Autodesk Inventor part; units mm, degrees
ref_plane "YZ Plane" through (0, 0, 0) normal (1, 0, 0) x (0, 1, 0)
ref_plane "XZ Plane" through (0, 0, 0) normal (0, 1, 0) x (-1, 0, 0)
ref_plane "XY Plane" through (0, 0, 0) normal (0, 0, 1) x (1, 0, 0)
sketch "Sketch_1" plane through (0, 0, 0) normal (0, 0, 1) x (1, 0, 0)
  line L0 (11, 0) -> (-2.8, 0)
  line L1 (-2.8, 0) -> (-2.8, 5)
  line L2 (-2.8, 5) -> (0, 5)
  line L3 (0, 5) -> (0, 3)
  line L4 (0, 3) -> (11, 3)
  line L5 (11, 3) -> (11, 0)
  line L6 (11, 0) -> (-2.8, 0)
revolve "Revolution1" add sketch "Sketch_1" angle 360 about axis through (11, 0, 0) along (1, 0, 0)
sketch "Sketch2" plane through (-2.8, 0, 0) normal (-1, 0, 0) x (0, 0, 1)
  point P0 (0, 0)
hole "Hole1" at (-2.8, 0, 0) direction (1, 0, 0) diameter 2.5 depth 2.5 tip angle 120
sketch "Sketch_3" plane through (-2.8, 0, 0) normal (1, 0, 0) x (0, 0, -1)
  line L0 (-1.25, -0.7217) -> (0, -1.4434)
  line L1 (0, -1.4434) -> (1.25, -0.7217)
  line L2 (1.25, -0.7217) -> (1.25, 0.7217)
  line L3 (1.25, 0.7217) -> (0, 1.4434)
  line L4 (0, 1.4434) -> (-1.25, 0.7217)
  line L5 (-1.25, 0.7217) -> (-1.25, -0.7217)
extrude "Extrusion1" cut sketch "Sketch_3" along normal blind 2.5
sketch "Sketch_6" plane through (0, 0, 0) normal (0, 0, 1) x (1, 0, 0)
  line L0 (19, 0) -> (11, 0)
  line L1 (11, 0) -> (11, 2)
  line L2 (11, 2) -> (18.5705, 2)
  line L3 (18.5705, 2) -> (19, 1.5705)
  line L4 (19, 1.5705) -> (19, 0)
  line L5 (19, 0) -> (11, 0)
revolve "Revolution2" add sketch "Sketch_6" angle 360 about axis through (19, 0, 0) along (1, 0, 0)
thread "Thread1"
properties part number "DBTS4-11-8"
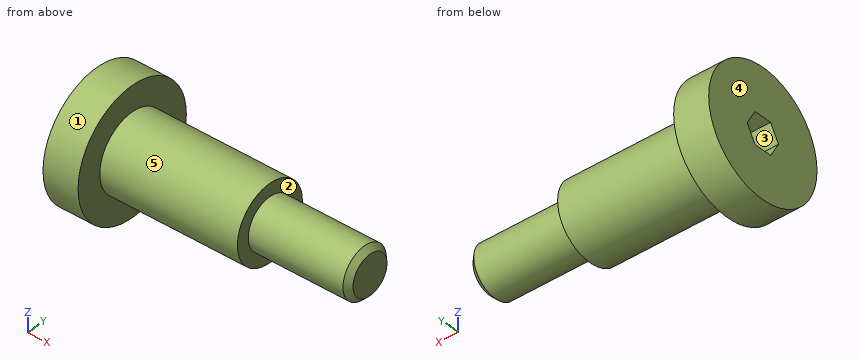
Input: part model. Units: mm. Frame: model coordinates. Face numbers are marked on the shaded views. A direction names the side the tool comes from. Give positions to 0.01 mm unless a question says otherwise; leave off trailing zeros. Write each loop counter-clockwise with the first axis right and the second up, starting at its lowest first coordinate (ties: lowest second). Pieces come first, ordered by that corner, then holes. Notation, with made-up numbers: (25, -27) - (81, -27) arc R35 ccw to (81, 9) - close; hole circle Ø2 at (-2, 25.25). An arc over 180 degrees is marked (long way). Write item = value, one per line. Start each with the question number.
1) Cut plane B-B (x = 10.5). Return loops of the section in (y, z).
2) Pin query (flat end, axial travel): pin 1 (3 mm diameter, centred on x = 8, y = -2.5, fed in from -Z); pin 2 (6 mm diameter, centred on x = 10.5, y = -1.5, fed in from +Z); pin 3 (2 mm diameter, centred on x = 11.5, z = 0.5, fed in from +Y). Return the tip coordinate at first contact, or that it passes through.
3) Draft query along Z for the marked faces 3, 4 and 5. Return one class per face: pulls with the +Z half, pulls with the -Z half, needs draft (parallel to the pull), parting line crosses it, or undercut.
4) Cut plane C-C (y = 3.5). Return loops of the section in (x, z).
5) Cut plane D-D (z = 4.25). Return loops of the section in (x, y), and give its area (3 significant figures).
6) Reachability of the marked faces 1 and 2 from +Z, -Z, +X, -X, +Y, -Y: full face, straight path, thin tool, end or side. Return the list, or none.
7) Cut plane A-A (z = -2.75). Return loops of the section in (x, y), and give its area (3 significant figures).
8) Material intervals for L1, parallel to X at y = -1.25, z = 4; L2, parallel to Z at x = 12, y = 0; L3, parallel to X at y = -1, z = 2, sorted ascending. Write a range as [from, to].
Answers follow:
q1.outline = circle Ø6 at (0, 0)
q2.pin_1 = -2.83
q2.pin_2 = 3
q2.pin_3 = 3
q3.face_3 = undercut
q3.face_4 = needs draft
q3.face_5 = parting line crosses it
q4.outline = (-2.8, -3.57) - (0, -3.57) - (0, 3.57) - (-2.8, 3.57) - close
q5.outline = (-2.8, -2.63) - (0, -2.63) - (0, 2.63) - (-2.8, 2.63) - close
q5.area = 14.7 mm^2
q6.face_1 = +X, -X
q6.face_2 = +X
q7.outline = (-2.8, -4.18) - (0, -4.18) - (0, -1.2) - (11, -1.2) - (11, 1.2) - (0, 1.2) - (0, 4.18) - (-2.8, 4.18) - close
q7.area = 49.8 mm^2
q8.L1 = [-2.8, 0]
q8.L2 = [-2, 2]
q8.L3 = [-2.8, 11]
